```python
from build123d import *

# Parameters (mm, degrees)
SKETCH1_R                       = 7.5
BOSS_EXTRUDE1_DEPTH             = 8.5
CUT_EXTRUDE1_DEPTH              = 6.8
SKETCH3_R                       = 1.5
CUT_EXTRUDE2_DEPTH              = 16.249262277
FILLET1_R                       = 1.5
SKETCH5_R                       = 6
BOSS_EXTRUDE3_DEPTH             = 21.3
BOSS_EXTRUDE3_DIRECTION_2_REACH = 33.631
FILLET1_OF_MIRROR1_R            = 1.5


with BuildPart() as part:
    # Sketch1 → Boss-Extrude1 (new body)
    with BuildSketch(Plane.XY):
        Circle(SKETCH1_R)
    boss_extrude1 = extrude(amount=BOSS_EXTRUDE1_DEPTH)

    # Sketch2 → Cut-Extrude1 (cut)
    with BuildSketch(Plane.XY.offset(8.5)):
        Polygon((2.7, 0), (2.7, 13.78279584), (-2.7, 13.78279584), (-2.7, 0), (-2.7, -14.12853377), (2.7, -14.12853377), align=None)
    cut_extrude1 = extrude(amount=-CUT_EXTRUDE1_DEPTH, mode=Mode.SUBTRACT)

    # Sketch3 → Cut-Extrude2 (cut, symmetric)
    with BuildSketch(Plane(origin=(-2.7, 0, 0), x_dir=(0, 0, -1), z_dir=(1, 0, 0))):
        with Locations(Location((-5.3, 0, 0), (0, 0, 180))):
            Circle(SKETCH3_R)
    cut_extrude2 = extrude(amount=CUT_EXTRUDE2_DEPTH, both=True, mode=Mode.SUBTRACT)

    # Fillet1
    fillet1_edges = [part.edges().sort_by_distance(p)[0] for p in [
        (-2.7, 0, 1.7),
        (2.7, 0, 1.7),
        (2.7, 0, 8.5),
        (-2.7, 0, 8.5),
    ]]
    fillet(fillet1_edges, radius=FILLET1_R)

    # Sketch5 → Boss-Extrude3 (add)
    with BuildSketch(Plane(origin=(0, 0, -21.3), x_dir=(-1, 0, 0), z_dir=(0, 0, -1))):
        Circle(SKETCH5_R)
    extrude(amount=BOSS_EXTRUDE3_DEPTH)

    # Sketch5 → Boss-Extrude3 direction 2 (add, up to next)
    with BuildSketch(Plane(origin=(0, 0, -21.3), x_dir=(-1, 0, 0), z_dir=(0, 0, -1)), mode=Mode.PRIVATE) as boss_extrude3_direction_2_sk1:
        Circle(SKETCH5_R)
    boss_extrude3_direction_2_tool1 = extrude(boss_extrude3_direction_2_sk1.sketch, amount=-BOSS_EXTRUDE3_DIRECTION_2_REACH, mode=Mode.PRIVATE) - part.part
    add(boss_extrude3_direction_2_tool1.solids().sort_by_distance((0, 0, -21.3))[0])

    # Mirror1: Boss-Extrude1, Cut-Extrude1, Cut-Extrude2 across plane
    add(boss_extrude1.mirror(Plane(origin=(0, 0, -21.3), x_dir=(1, 0, 0), z_dir=(0, 0, -1))))
    add(cut_extrude1.mirror(Plane(origin=(0, 0, -21.3), x_dir=(1, 0, 0), z_dir=(0, 0, -1))), mode=Mode.SUBTRACT)
    add(cut_extrude2.mirror(Plane(origin=(0, 0, -21.3), x_dir=(1, 0, 0), z_dir=(0, 0, -1))), mode=Mode.SUBTRACT)

    # Fillet1 of Mirror1
    fillet1_of_mirror1_edges = [part.edges().sort_by_distance(p)[0] for p in [
        (-2.7, 0, -44.3),
        (2.7, 0, -44.3),
        (2.7, 0, -51.1),
        (-2.7, 0, -51.1),
    ]]
    fillet(fillet1_of_mirror1_edges, radius=FILLET1_OF_MIRROR1_R)


solid = part.part
```
Work out the finished part from the listing and answer in its coordinate system (mm). A direction names the side the tool comes from. Give positions to 0.01 mm unless a question says otherwise; leave off trailing zeros. Loops run counter-clockwise (first coordinate to the right, second up) from the corner with the lowest first, then second, coordinate; pieces in that order, holes last. Notation, with made-up numbers: (84.5, -13) - (132.5, -13) arc R32 cw to (132.5, 23) - close; hole circle Ø2 at (-8.75, 68). An arc over 180 degrees is marked (long way). One line per question, with ' | ' between items.
(1) The part is cut by section D-D (x = -4.75). Write down the section's boundary in (y, z).
Recorded:
outline: (-5.8, -51.1) - (5.8, -51.1) - (5.8, -42.6) - (3.67, -42.6) - (3.67, 0) - (5.8, 0) - (5.8, 8.5) - (-5.8, 8.5) - (-5.8, 0) - (-3.67, 0) - (-3.67, -42.6) - (-5.8, -42.6) - close; hole circle Ø3 at (0, -47.9); hole circle Ø3 at (0, 5.3)
(2) A tool of negligible diameter and unlimited length cuts with its end or side. For faces 4 (the face through (3.15, 0.1, 8.07)), 5 (the face through (2.7, -2, -48)), 6 (the face through (5, 0, -51.1)), from which of +Z, -Z, +X, -X, +Y, -Y can it reach the whole face along a straight path? Write none if from no direction.
Recorded:
face 4: +Z, +Y, -Y | face 5: -Z, +Y, -Y | face 6: -Z, +X, -X, +Y, -Y
(3) Each of these flat-tipped pins is pushed along its axis until it touches: pin 1 Ø3 at (x, z) = (3, 1.5) entering from +Y; pin 2 Ø2.5 at (y, z) = (0, -47.9) entering from +X; pin 3 Ø1.5 at (x, z) = (-3, -42) entering from +Y; pin 4 Ø6 at (x, z) = (2.5, -14.5) entering from -Y. Where does it stop, or does it pass through?
Recorded:
pin 1: stops at y = 7.35 | pin 2: passes through | pin 3: stops at y = 7.05 | pin 4: stops at y = -6
(4) The part is cut by section C-C (y = 0). Count the separate pieces of the cut face and the enclosed holes in it, then the cut area to 3 significant figures.
Recorded:
separate pieces: 5 | enclosed holes: 0 | area: 635 mm²
(5) The part is cut by section A-A (z = 5.3). Write down the section's boundary in (x, y).
Recorded:
outline: (-7.35, -1.5) arc R7.5 ccw to (-2.7, -7) - (-2.7, -1.5) - close; (-7.35, 1.5) - (-2.7, 1.5) - (-2.7, 7) arc R7.5 ccw to start; (2.7, -7) arc R7.5 ccw to (7.35, -1.5) - (2.7, -1.5) - close; (2.7, 1.5) - (7.35, 1.5) arc R7.5 ccw to (2.7, 7) - close
(6) Straight lines are drawn through the part: probe 1 along Z at (x, y) = (5.5, 4); probe 2 along X at (y, z) = (0, -46); probe 3 along Z at (x, y) = (1, -2). For each, find the intervals that lie inside material, in ascending order.
Recorded:
probe 1: z = -51.1 to -42.6, 0 to 8.5 | probe 2: x = -7.5 to -2.7, 2.7 to 7.5 | probe 3: z = -44.3 to 1.7
(7) The part is cut by section B-B (x = 0). Write down the section's boundary in (y, z).
Recorded:
outline: (-7.5, -44.3) - (7.5, -44.3) - (7.5, -42.6) - (6, -42.6) - (6, 0) - (7.5, 0) - (7.5, 1.7) - (-7.5, 1.7) - (-7.5, 0) - (-6, 0) - (-6, -42.6) - (-7.5, -42.6) - close
(8) The mould has two halves that part along Y. Classify faces 1 (the face through (7.154, 2.253, -46.79)), 2 (the face through (2, 6, 0)), 3 (the face through (-5.07, -0.45, -49.33)): +Y half, -Y half, draft (parallel to the pull), parting line (faces both ways), or undercut.
Recorded:
face 1: parting line | face 2: draft | face 3: undercut
